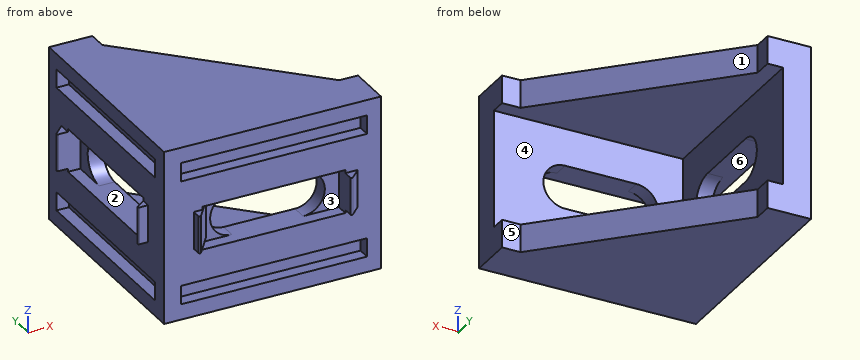
from build123d import *

# Parameters (mm, degrees)
SKETCH1_W           = 35
SKETCH1_H           = 28
BOSS_EXTRUDE1_DEPTH = 4.5
BOSS_EXTRUDE2_DEPTH = 4.5
SKETCH3_W           = 19
SKETCH3_H           = 30.5
BOSS_EXTRUDE3_DEPTH = 4.5
CUT_EXTRUDE1_DEPTH  = 4.5
SKETCH5_W           = 7
SKETCH5_H           = 23
SKETCH5_W_2         = 3
SKETCH5_H_2         = 30
CUT_EXTRUDE2_DEPTH  = 2
BOSS_EXTRUDE4_DEPTH = 3


with BuildPart() as part:
    # Sketch1 → Boss-Extrude1 (new body)
    with BuildSketch(Plane(origin=(0, 0, 0), x_dir=(1, 0, 0), z_dir=(0, 1, 0))):
        Rectangle(SKETCH1_W, SKETCH1_H)
        with BuildLine():
            Line((-5.5, 3.5), (6, 3.5))
            ThreePointArc((6, 3.5), (9.5, 0), (6, -3.5))
            Line((6, -3.5), (-5.5, -3.5))
            ThreePointArc((-5.5, -3.5), (-9, 0), (-5.5, 3.5))
        make_face(mode=Mode.SUBTRACT)
    extrude(amount=BOSS_EXTRUDE1_DEPTH)

    # Sketch2 → Boss-Extrude2 (add)
    with BuildSketch(Plane.XY.offset(14)):
        Polygon((17.5, 4.5), (17.5, 7), (14.5, 7), (-10.5, 32), (-10.5, 35), (-17.5, 35), (-17.5, 4.5), align=None)
    boss_extrude2 = extrude(amount=-BOSS_EXTRUDE2_DEPTH)

    # Mirror1: Boss-Extrude2 across plane
    add(boss_extrude2.mirror(Plane.XY))

    # Sketch3 → Boss-Extrude3 (add)
    with BuildSketch(Plane.ZY.offset(17.5)):
        with Locations((0, 19.75)):
            Rectangle(SKETCH3_W, SKETCH3_H)
    extrude(amount=-BOSS_EXTRUDE3_DEPTH)

    # Sketch4 → Cut-Extrude1 (cut)
    with BuildSketch(Plane.ZY.offset(17.5)):
        with BuildLine():
            Line((3.5, 23.5), (3.5, 12))
            ThreePointArc((3.5, 12), (0, 8.5), (-3.5, 12))
            Line((-3.5, 12), (-3.5, 23.5))
            ThreePointArc((-3.5, 23.5), (0, 27), (3.5, 23.5))
        make_face()
    cut_extrude1 = extrude(amount=-CUT_EXTRUDE1_DEPTH, mode=Mode.SUBTRACT)

    # Sketch5 → Cut-Extrude2 (cut)
    with BuildSketch(Plane.ZY.offset(17.5)):
        with Locations((0, 17.75)):
            Rectangle(SKETCH5_W, SKETCH5_H)
        with Locations((-10, 17.75)):
            Rectangle(SKETCH5_W_2, SKETCH5_H_2)
        with Locations((10, 17.75)):
            Rectangle(SKETCH5_W_2, SKETCH5_H_2)
    cut_extrude2 = extrude(amount=-CUT_EXTRUDE2_DEPTH, mode=Mode.SUBTRACT)

    # Sketch6 → Boss-Extrude4 (add, symmetric)
    with BuildSketch(Plane.XY):
        with BuildLine():
            Line((-17.5, 4.8), (-18.9, 4.8))
            ThreePointArc((-18.9, 4.8), (-19.08973666, 4.936754447), (-19.02, 5.16))
            Line((-19.02, 5.16), (-15.5, 7.8))
            Line((-15.5, 7.8), (-15.5, 4.8))
            Line((-15.5, 4.8), (-17.5, 4.8))
        make_face()
        with BuildLine():
            Line((-17.5, 29.25), (-19.017157288, 29.25))
            ThreePointArc((-19.017157288, 29.25), (-19.201933194, 29.373463314), (-19.158578644, 29.591421356))
            Line((-19.158578644, 29.591421356), (-17.5, 31.25))
            Line((-17.5, 31.25), (-17.5, 29.25))
        make_face()
    boss_extrude4 = extrude(amount=BOSS_EXTRUDE4_DEPTH, both=True)

    # Mirror2: Cut-Extrude1, Cut-Extrude2, Boss-Extrude4 across plane
    add(cut_extrude1.mirror(Plane(origin=(-8.75, 8.75, 0), x_dir=(0, 0, 1), z_dir=(-0.7071067811865475, 0.7071067811865477, 0))), mode=Mode.SUBTRACT)
    add(cut_extrude2.mirror(Plane(origin=(-8.75, 8.75, 0), x_dir=(0, 0, 1), z_dir=(-0.7071067811865475, 0.7071067811865477, 0))), mode=Mode.SUBTRACT)
    add(boss_extrude4.mirror(Plane(origin=(-8.75, 8.75, 0), x_dir=(0, 0, 1), z_dir=(-0.7071067811865475, 0.7071067811865477, 0))))


solid = part.part
Input: part model. Units: mm. Frame: model coordinates. Face numbers are marked on the shaded views. A direction names the side the tool comes from. Give positions to 0.01 mm unless a question says otherwise; leave off trailing zeros. Order: outer loops, then holes, each group sorted by start corner. A loop starts at its lowest first (then second) coordinate and runs counter-clockwise, first axis right, second up. Notation, with made-up numbers: (-19, 77.5) - (27, 77.5) arc R27 cw to (27, 93.5) - close; hole circle Ø10 at (-14, -7.5). An arc over 180 degrees is marked (long way). Answer as a JSON object with one key per item and string values. Group by question number.
Q1. Cut plane C-C, the plane y = 14.5. Output: boundary loops of the cut face in (x, z), then the cut area to 4 significant figures.
Q2. Cut plane D-D, the plane y = 4. Output: boundary loops of the cut face in (x, z).
Q3. Cut plane B-B, the plane x = 1. Output: boundary loops of the cut face in (y, z), then the cut area to 4 significant figures.
Q4. Line query: probe 1 along Z at (x, y) = (2, 0.5); probe 2 along Z at (x, y) = (-5.5, 7.5); probe 3 along Z at (x, y) = (-15, 15.5). Output: solid intervals per line, ascending.
Q5. Set-up query: the marked faces 4, 5 and 6. Return all of +Z, -Z, +X, -X, +Y, -Y with unobstructed straight access to the full face (end or side cutting, diameter ignored); none if empty.
Q6. Mould query, pull axis X, two halves, no side actions, for the marked faces 1, 2 and 3. Classes: pulls with the +X half, pulls with the -X half, needs draft (parallel to the pull), parting line crosses it, or undercut.
Q7. First-contact query: pin 1 Ø2.5 at (y, z) = (34, -10.5) entering from +X; pin 2 Ø1 at (y, z) = (30, -6.5) entering from +X; pin 3 Ø5.5 at (x, z) = (-4.5, -1) entering from +Y. Flat tips, straight axial feed; report the tip coordinate or a pass-through.
Q8. Cut plane A-A, the plane z = 0. Count the separate pieces of the cut face and the enclosed holes in it, then the cut area to 3 significant figures.
Results:
{
 "1": {"outline": "(-17.5, -14) - (7, -14) - (7, -9.5) - (-13, -9.5) - (-13, -3.5) - (-17.5, -3.5) - (-17.5, -8.5) - (-15.5, -8.5) - (-15.5, -11.5) - (-17.5, -11.5) - close; (-17.5, 3.5) - (-13, 3.5) - (-13, 9.5) - (7, 9.5) - (7, 14) - (-17.5, 14) - (-17.5, 11.5) - (-15.5, 11.5) - (-15.5, 8.5) - (-17.5, 8.5) - close", "area": "262.5 mm^2"},
 "2": {"outline": "(-17.5, -14) - (17.5, -14) - (17.5, 14) - (-17.5, 14) - (-17.5, 11.5) - (-15.5, 11.5) - (-15.5, 8.5) - (-17.5, 8.5) - (-17.5, -8.5) - (-15.5, -8.5) - (-15.5, -11.5) - (-17.5, -11.5) - close; hole (-5.5, -3.5) - (6, -3.5) arc R3.5 ccw to (6, 3.5) - (-5.5, 3.5) arc R3.5 ccw to start"},
 "3": {"outline": "(0, -14) - (20.5, -14) - (20.5, -9.5) - (4.5, -9.5) - (4.5, -3.5) - (0, -3.5) - (0, -8.5) - (2, -8.5) - (2, -11.5) - (0, -11.5) - close; (0, 3.5) - (4.5, 3.5) - (4.5, 9.5) - (20.5, 9.5) - (20.5, 14) - (0, 14) - (0, 11.5) - (2, 11.5) - (2, 8.5) - (0, 8.5) - close", "area": "226.5 mm^2"},
 "4": {"probe 1": "-14 to -11.5, -8.5 to -3.5, 3.5 to 8.5, 11.5 to 14", "probe 2": "-14 to -9.5, 9.5 to 14", "probe 3": "-14 to -3.5, 3.5 to 14"},
 "5": {"face 4": "+X, +Y", "face 5": "+Z, -Z, +X, +Y", "face 6": "-X"},
 "6": {"face 1": "pulls with the +X half", "face 2": "needs draft", "face 3": "undercut"},
 "7": {"pin 1": "x = -10.5", "pin 2": "x = -13", "pin 3": "y = 4.5"},
 "8": {"separate pieces": "3", "enclosed holes": "0", "area": "120 mm^2"}
}
